For this review, take the finished solid that the model builds, in its own axes (mm). Coordinates: 2 decimals unless noted, no trailing zeros. Write each loop counter-clockwise with the first axis right and the second up, starting at its lowest first coordinate (ties: lowest second). Pieces come first, ordered by that corner, then holes.
1) We need section A-A on z = 26. Write out the cut boundary in (x, y), then the cut area to 3 significant figures.
2) We need section D-D on x = 1.5. Write out the cut boundary in (y, z), then the cut area to 3 significant figures.
3) We need section B-B on z = 15.5. Write out the cut boundary in (x, y).
4) Insertion check: P1, Ø1.5, axis at x = 0, y = 0, coming from the -Z side; P2, Ø1.5, axis at x = 0, y = 0, coming from the +Z side. Each pin has a flat end and moves straight along its axis. Give the tip position at first contact, or say it passes through.
5) We need section C-C on y = 2.75. Write out the cut boundary in (x, z), then the cut area to 3 significant figures.
6) To check wall thickness, follow line 1 along X through (y, z) = (0, 25.75); line 2 along Y through (x, z) = (-0.6, 25.5); line 3 along Y through (x, z) = (2.1, 21.75). State the ranges of each line that lie inside material, in increasing order.
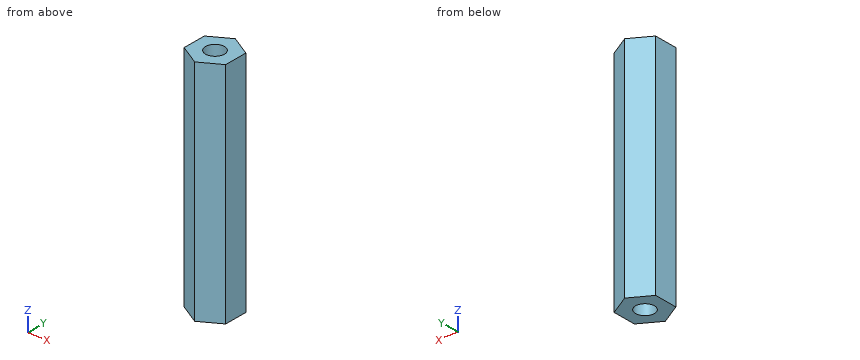
from build123d import *

# Parameters (mm, degrees)
BOSS_EXTRU_1_DEPTH                            = 30
TROU_POUR_TARAUDAGE_POUR_TROU_TARAUD_M3_D     = 2.5
TROU_POUR_TARAUDAGE_POUR_TROU_TARAUD_M3_DEPTH = 7
TROU_POUR_TARAUDAGE_POUR_TROU_TARAUD_M3_TIP   = 0.751075774
TROU_POUR_TARAUDAGE_POUR_TROU_TARAUD_2_D      = 2.5
TROU_POUR_TARAUDAGE_POUR_TROU_TARAUD_2_DEPTH  = 7
TROU_POUR_TARAUDAGE_POUR_TROU_TARAUD_2_TIP    = 0.751075774


with BuildPart() as part:
    # Esquisse1 → Boss.-Extru.1 (new body)
    with BuildSketch(Plane.XY):
        Polygon((0, -3.175426481), (2.75, -1.58771324), (2.75, 1.58771324), (0, 3.175426481), (-2.75, 1.58771324), (-2.75, -1.58771324), align=None)
    extrude(amount=BOSS_EXTRU_1_DEPTH)

    # Trou pour taraudage pour trou taraud_ M3
    with Locations(Plane.XY.offset(30)):
        with Locations((0, 0)):
            Hole(TROU_POUR_TARAUDAGE_POUR_TROU_TARAUD_M3_D / 2, depth=TROU_POUR_TARAUDAGE_POUR_TROU_TARAUD_M3_DEPTH)
            with Locations((0, 0, -(TROU_POUR_TARAUDAGE_POUR_TROU_TARAUD_M3_DEPTH + TROU_POUR_TARAUDAGE_POUR_TROU_TARAUD_M3_TIP / 2))):  # 118° drill point
                Cone(0, TROU_POUR_TARAUDAGE_POUR_TROU_TARAUD_M3_D / 2, TROU_POUR_TARAUDAGE_POUR_TROU_TARAUD_M3_TIP, mode=Mode.SUBTRACT)

    # Trou pour taraudage pour trou taraud 2
    with Locations(Plane(origin=(0, 0, 0), x_dir=(-1, 0, 0), z_dir=(0, 0, -1))):
        with Locations((0, 0)):
            Hole(TROU_POUR_TARAUDAGE_POUR_TROU_TARAUD_2_D / 2, depth=TROU_POUR_TARAUDAGE_POUR_TROU_TARAUD_2_DEPTH)
            with Locations((0, 0, -(TROU_POUR_TARAUDAGE_POUR_TROU_TARAUD_2_DEPTH + TROU_POUR_TARAUDAGE_POUR_TROU_TARAUD_2_TIP / 2))):  # 118° drill point
                Cone(0, TROU_POUR_TARAUDAGE_POUR_TROU_TARAUD_2_D / 2, TROU_POUR_TARAUDAGE_POUR_TROU_TARAUD_2_TIP, mode=Mode.SUBTRACT)


solid = part.part
Result:
1. outline: (-2.75, -1.59) - (0, -3.18) - (2.75, -1.59) - (2.75, 1.59) - (0, 3.18) - (-2.75, 1.59) - close; hole circle Ø2.5 at (0, 0)
1. area: 21.3 mm2
2. outline: (-2.31, 0) - (2.31, 0) - (2.31, 30) - (-2.31, 30) - close
2. area: 139 mm2
3. outline: (-2.75, -1.59) - (0, -3.18) - (2.75, -1.59) - (2.75, 1.59) - (0, 3.18) - (-2.75, 1.59) - close
4. P1: stops at z = 7.3
4. P2: stops at z = 22.7
5. outline: (-0.74, 0) - (0.74, 0) - (0.74, 30) - (-0.74, 30) - close
5. area: 44.2 mm2
6. line 1: x = -2.75 to -1.25, 1.25 to 2.75
6. line 2: y = -2.83 to -1.1, 1.1 to 2.83
6. line 3: y = -1.96 to 1.96
